```python
from build123d import *

# Parameters (mm, degrees)
F0_W     = 20.0025
F0_H     = 28.9941
F1_DEPTH = 21.9964
F2_SIZE  = 10.0076


with BuildPart() as f1:
    # F0 (on Front) → F1 (new body)
    with BuildSketch(Plane.XZ):
        with Locations((10.00125, -14.49705)):
            Rectangle(F0_W, F0_H)
        with BuildLine():
            Line((0, 4.9911), (0, 0))
            Line((0, 0), (20.0025, 0))
            Line((20.0025, 0), (20.0025, 28.9941))
            Line((20.0025, 28.9941), (0, 28.9941))
            Line((0, 28.9941), (0, 18.9865))
            ThreePointArc((0, 18.9865), (4.948121, 16.936921), (6.9977, 11.9888))
            ThreePointArc((6.9977, 11.9888), (4.948121, 7.040679), (0, 4.9911))
        make_face()
        with BuildLine():
            Line((-20.0025, 0), (0, 0))
            Line((0, 0), (0, 4.9911))
            ThreePointArc((0, 4.9911), (-6.9977, 11.9888), (0, 18.9865))
            Line((0, 18.9865), (0, 28.9941))
            Line((0, 28.9941), (-20.0025, 28.9941))
            Line((-20.0025, 28.9941), (-20.0025, 0))
        make_face()
        with Locations((-10.00125, -14.49705)):
            Rectangle(F0_W, F0_H)
    extrude(amount=F1_DEPTH)

    # F2
    f2_edges = [f1.edges().sort_by_distance(p)[0] for p in [
        (20.0025, -10.9982, 28.9941),
        (-20.0025, -10.9982, 28.9941),
    ]]
    chamfer(f2_edges, length=F2_SIZE)


solid = f1.part
```
Source: CAD feature listing. Evaluate the final solid. Frame: model axes, mm. Coordinates: 2 decimals unless noted, no trailing zeros. Loops run counter-clockwise (first coordinate to the right, second up) from the corner with the lowest first, then second, coordinate; pieces in that order, holes last. Notation, with made-up numbers: (38, -11.5) - (90, -11.5) arc R8 ccw to (90, -0.5) - close; hole circle Ø7 at (4, -5.5). An arc over 180 degrees is marked (long way). Answer as CSV lines item,"result".
1. Contact query for a flat-ended pin moving along its axis: pin 1 (8 mm diameter, centred on x = -4, z = 12.5, fed in from +Y). Output: stop coordinate, or through.
Established:
pin 1,"stops at y = 0"
2. Section B-B (x = 4.5). Return loops of the section in (y, z).
Established:
outline,"(-22, -28.99) - (0, -28.99) - (0, 6.63) - (-22, 6.63) - close; (-22, 17.35) - (0, 17.35) - (0, 28.99) - (-22, 28.99) - close"
3. Ray query, line 1 (Z direction, x = 0, y = -8.5); line 2 (Z direction, x = 4.5, y = -4.75); line 3 (X direction, y = -7.25, z = 8.5). Return the intervals inside material, ascending.
Established:
line 1,"z = -28.99 to 4.99, 18.99 to 28.99"
line 2,"z = -28.99 to 6.63, 17.35 to 28.99"
line 3,"x = -20 to -6.07, 6.07 to 20"
4. Section C-C (x = -4). Return loops of the section in (y, z), then the cut area to 3 significant figures.
Established:
outline,"(-22, -28.99) - (0, -28.99) - (0, 6.25) - (-22, 6.25) - close; (-22, 17.73) - (0, 17.73) - (0, 28.99) - (-22, 28.99) - close"
area,"1,020 mm2"
5. Section A-A (y = -3.5). Return loops of the section in (x, z), then the cut area to 3 significant figures.
Established:
outline,"(-20, -28.99) - (20, -28.99) - (20, 18.99) - (9.99, 28.99) - (-9.99, 28.99) - (-20, 18.99) - close; hole circle Ø14 at (0, 11.99)"
area,"2,070 mm2"
